Study the drawing (mm; zero at the part's minimum x, y, z) and answer. A direction names the side the tool comes from. Round coordinates to 2 decimals unless told otherwise and drop trailing zeros. Order: outer loops, then holes, each group sorted by start corner. A loop starts at its lowest first (then second) coordinate and runs counter-clockwise, first axis right, second up. Notation, with made-up numbers: (-37.5, 50.5) - (6.5, 50.5) arc R14 ccw to (6.5, 66.5) - close; hole circle Ø7 at (46.5, -22). An arc over 180 degrees is marked (long way). Put each result on its own line as item: value. Start each with the question number.
Q1. Section D-D on y = 10.5 is taken. Give the vertices of the cut face in (x, z).
Q2. Find the intervals of material crossed by line 1 along Z through (x, y) = (5.2, 6); line 2 along Z through (x, y) = (2, 10.25); line 3 along Z through (x, y) = (6.5, 2.75), in increasing order. Write a range as from..to.
Q3. Which of the six approach directions +Z, -Z, +X, -X, +Y, -Y give full straight-line access (tool end or side, diameter ignored) to the marked faces 1, 2 and 3?
Q4. Section C-C on x = 5.75 is taken. Give the vertices of the cut face in (y, z).
Q5. Section B-B on y = 6 is taken. Give the vertices of the cut face in (x, z), then the cut area to 3 significant figures.
Q6. Each of these flat-tipped pins is pushed along its axis until it touches: pin 1 Ø3 at (y, z) = (6, 28) entering from -X; pin 2 Ø6 at (y, z) = (7, 28) entering from -X; pin 3 Ø0.8 at (x, y) = (2.5, 3) entering from +Z; pin 4 Ø3 at (y, z) = (5, 11) entering from +X. Where does it stop, or does it pass through?
Q7. Section A-A on z = 28 is taken. Give the vertices of the cut face in (x, y), then the cut area to 3 significant figures.
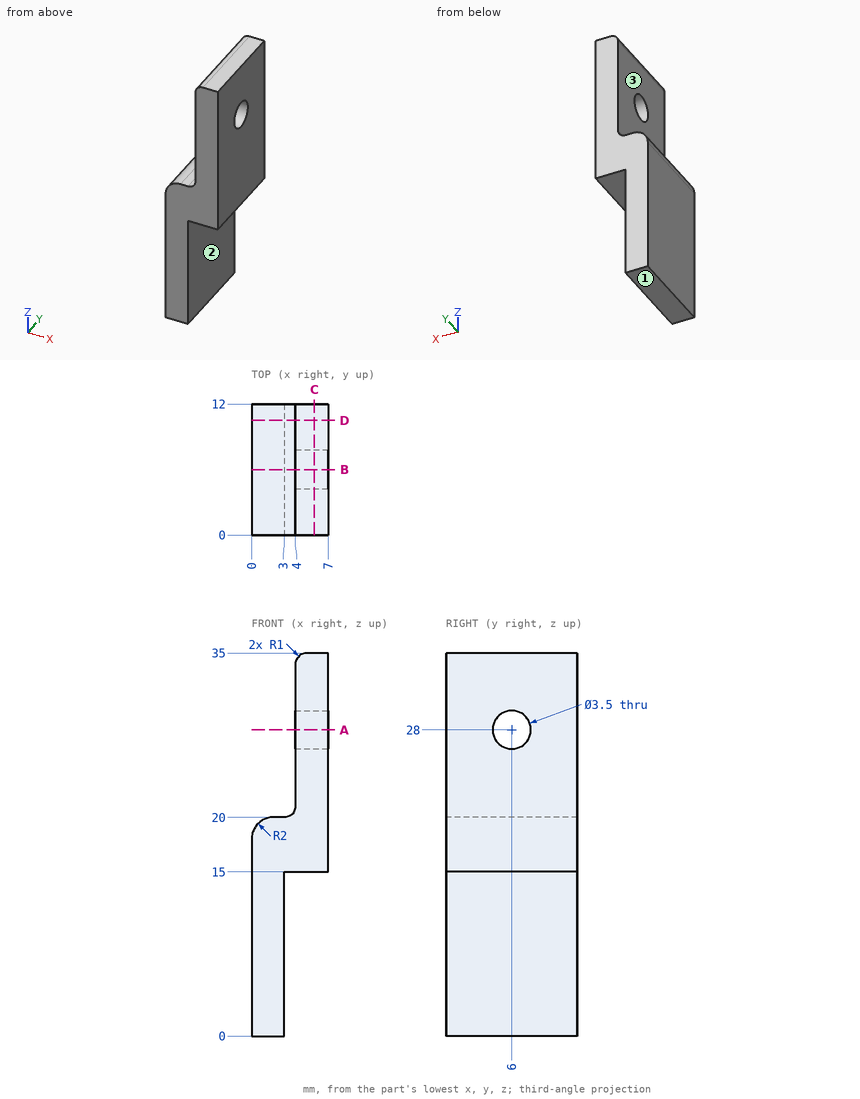
Findings:
1. outline: (0, 0) - (3, 0) - (3, 15) - (7, 15) - (7, 35) - (5, 35) arc R1 ccw to (4, 34) - (4, 21) arc R1 cw to (3, 20) - (2, 20) arc R2 ccw to (0, 18) - close
2. line 1: 15..26.25, 29.75..35
2. line 2: 0..20
2. line 3: 15..35
3. face 1: -Z, +X, -X, +Y, -Y
3. face 2: -Z, +X, +Y, -Y
3. face 3: +Z, -X, +Y, -Y
4. outline: (0, 15) - (12, 15) - (12, 35) - (0, 35) - close; hole circle Ø3.5 at (6, 28)
5. outline: (0, 0) - (3, 0) - (3, 15) - (7, 15) - (7, 26.25) - (4, 26.25) - (4, 21) arc R1 cw to (3, 20) - (2, 20) arc R2 ccw to (0, 18) - close; (4, 29.75) - (7, 29.75) - (7, 35) - (5, 35) arc R1 ccw to (4, 34) - close
5. area: 114 mm2
6. pin 1: through
6. pin 2: x = 4
6. pin 3: z = 20
6. pin 4: x = 3
7. outline: (4, 0) - (7, 0) - (7, 4.25) - (4, 4.25) - close; (4, 7.75) - (7, 7.75) - (7, 12) - (4, 12) - close
7. area: 25.5 mm2
